Could you check a few things on this model? Use its own coordinates, in mm. A direction names the side the tool comes from. Coordinates: 2 decimals unless noted, no trailing zeros. Write each loop counter-clockwise with the first axis right and the second up, starting at its lowest first coordinate (ties: lowest second). Pieces come first, ordered by that corner, then holes.
```python
from build123d import *

# Parameters (mm, degrees)
EXTRUDE_1_DEPTH             = 90
SKETCH_2_W                  = 90
SKETCH_2_H                  = 17.75
EXTRUDE_2_DEPTH             = 8.2
SKETCH_3_W                  = 90
SKETCH_3_H                  = 50.95
EXTRUDE_3_DEPTH             = 8.2
SKETCH_4_W                  = 3.95
SKETCH_4_H                  = 29.5
CUT_EXTRUDE_1_DEPTH         = 96.44153315
SKETCH_5_W                  = 3.95
SKETCH_5_H                  = 6.2
CUT_EXTRUDE_2_DEPTH         = 96.44153315
SKETCH_6_W                  = 2.25
SKETCH_6_H                  = 3.95
CUT_EXTRUDE_3_DEPTH         = 96.44153315
SKETCH_7_W                  = 4.5
SKETCH_7_H                  = 3.95
CUT_EXTRUDE_4_DEPTH         = 96.44153315
SKETCH_8_W                  = 2.25
SKETCH_8_H                  = 3.95
CUT_EXTRUDE_5_DEPTH         = 96.44153315
SKETCH_9_W                  = 3.95
SKETCH_9_H                  = 2.25
CUT_EXTRUDE_6_DEPTH         = 96.44153315
SKETCH_10_W                 = 20.2
SKETCH_10_H                 = 45.2
CUT_EXTRUDE_7_DEPTH         = 86
HOLE_WIZARD_2_5_2_5_1_D     = 2.5
HOLE_WIZARD_4_5_4_5_1_D     = 4.5
HOLE_WIZARD_8_3_8_3_1_D     = 8.3
HOLE_WIZARD_8_3_8_3_1_DEPTH = 3.2
FILLET_1_R                  = 2
FILLET_2_R                  = 2
EXTRUDE_START               = -90
SKETCH_17_R                 = 1.25
EXTRUDE_4_DEPTH             = 90
CUT_EXTRUDE_START           = -100
SKETCH_18_R                 = 4.15
CUT_EXTRUDE_8_DEPTH         = 100


with BuildPart() as part:
    # Эскиз1 → Бобышка-Вытянуть1 (new body)
    with BuildSketch(Plane(origin=(90, 0, 0), x_dir=(0, 0, -1), z_dir=(1, 0, 0))):
        with BuildLine():
            Line((6.75, -24.093761792), (6.75, 19.25))
            Line((6.75, 19.25), (-11.593761792, 19.25))
            ThreePointArc((-11.593761792, 19.25), (-15.325, 18), (-11.593761792, 16.75))
            Line((-11.593761792, 16.75), (-11, 16.75))
            Line((-11, 16.75), (-11, -16.75))
            Line((-11, -16.75), (-11.593761792, -16.75))
            ThreePointArc((-11.593761792, -16.75), (-15.325, -18), (-11.593761792, -19.25))
            Line((-11.593761792, -19.25), (-11, -19.25))
            Line((-11, -19.25), (-11, -23.5))
            Line((-11, -23.5), (-6.75, -23.5))
            Line((-6.75, -23.5), (-6.75, -24.093761792))
            ThreePointArc((-6.75, -24.093761792), (-5.5, -27.825), (-4.25, -24.093761792))
            Line((-4.25, -24.093761792), (-4.25, -23.5))
            Line((-4.25, -23.5), (4.25, -23.5))
            Line((4.25, -23.5), (4.25, -24.093761792))
            ThreePointArc((4.25, -24.093761792), (5.5, -27.825), (6.75, -24.093761792))
        make_face()
    extrude(amount=-EXTRUDE_1_DEPTH)

    # Эскиз2 → Бобышка-Вытянуть2 (add)
    with BuildSketch(Plane(origin=(0, 19.25, 0), x_dir=(-1, 0, 0), z_dir=(0, 1, 0))):
        with Locations((-45, 2.125)):
            Rectangle(SKETCH_2_W, SKETCH_2_H)
    extrude(amount=EXTRUDE_2_DEPTH)

    # Эскиз3 → Бобышка-Вытянуть3 (add)
    with BuildSketch(Plane(origin=(0, 0, -6.75), x_dir=(-1, 0, 0), z_dir=(0, 0, -1))):
        with Locations((-45, 1.975)):
            Rectangle(SKETCH_3_W, SKETCH_3_H)
    extrude(amount=EXTRUDE_3_DEPTH)

    # Эскиз4 → Вырез-Вытянуть1 (cut, through all)
    with BuildSketch(Plane.ZY):
        with Locations((-12.975, 0)):
            Rectangle(SKETCH_4_W, SKETCH_4_H)
    extrude(amount=-CUT_EXTRUDE_1_DEPTH, mode=Mode.SUBTRACT)

    # Эскиз5 → Вырез-Вытянуть2 (cut, through all)
    with BuildSketch(Plane.ZY):
        with Locations((-12.975, 24.35)):
            Rectangle(SKETCH_5_W, SKETCH_5_H)
    extrude(amount=-CUT_EXTRUDE_2_DEPTH, mode=Mode.SUBTRACT)

    # Эскиз6 → Вырез-Вытянуть3 (cut, through all)
    with BuildSketch(Plane.ZY):
        with Locations((-9.875, 25.475)):
            Rectangle(SKETCH_6_W, SKETCH_6_H)
    extrude(amount=-CUT_EXTRUDE_3_DEPTH, mode=Mode.SUBTRACT)

    # Эскиз7 → Вырез-Вытянуть4 (cut, through all)
    with BuildSketch(Plane.ZY):
        with Locations((0, 25.475)):
            Rectangle(SKETCH_7_W, SKETCH_7_H)
    extrude(amount=-CUT_EXTRUDE_4_DEPTH, mode=Mode.SUBTRACT)

    # Эскиз8 → Вырез-Вытянуть5 (cut, through all)
    with BuildSketch(Plane.ZY):
        with Locations((9.875, 25.475)):
            Rectangle(SKETCH_8_W, SKETCH_8_H)
    extrude(amount=-CUT_EXTRUDE_5_DEPTH, mode=Mode.SUBTRACT)

    # Эскиз9 → Вырез-Вытянуть6 (cut, through all)
    with BuildSketch(Plane.ZY):
        with Locations((-12.975, -22.375)):
            Rectangle(SKETCH_9_W, SKETCH_9_H)
    extrude(amount=-CUT_EXTRUDE_6_DEPTH, mode=Mode.SUBTRACT)

    # Эскиз10 → Вырез-Вытянуть7 (cut)
    with BuildSketch(Plane(origin=(90, 0, 0), x_dir=(0, 0, -1), z_dir=(1, 0, 0))):
        Rectangle(SKETCH_10_W, SKETCH_10_H)
    extrude(amount=-CUT_EXTRUDE_7_DEPTH, mode=Mode.SUBTRACT)

    # Диаметр отверстия Ø2.5 (2.5)1 (through all)
    with Locations(Plane(origin=(90, 0, 0), x_dir=(0, 0, -1), z_dir=(1, 0, 0))):
        with Locations((5.5, -25.75), (-13.25, -18), (-5.5, -25.75), (-13.25, 18)):
            Hole(HOLE_WIZARD_2_5_2_5_1_D / 2)

    # Диаметр отверстия Ø4.5 (4.5)1 (through all)
    with Locations(Plane.ZY):
        with Locations((-13.25, -18), (-13.25, 18), (-5.5, 25.75), (5.5, 25.75)):
            Hole(HOLE_WIZARD_4_5_4_5_1_D / 2)

    # Диаметр отверстия Ø8.3 (8.3)1
    with Locations(Plane.ZY):
        with Locations((0, 0)):
            Hole(HOLE_WIZARD_8_3_8_3_1_D / 2, depth=HOLE_WIZARD_8_3_8_3_1_DEPTH)

    # Скругление1
    fillet_1_edges = [part.edges().sort_by_distance(p)[0] for p in [
        (45, 23.5, 8.75),
    ]]
    fillet(fillet_1_edges, radius=FILLET_1_R)

    # Скругление2
    fillet_2_edges = [part.edges().sort_by_distance(p)[0] for p in [
        (45, 23.5, -8.75),
        (45, 23.5, 2.25),
        (45, 23.5, -2.25),
        (45, -21.25, -11),
        (4, 0, -10.1),
        (4, -22.6, 0),
        (4, 0, 10.1),
        (4, 22.6, 0),
        (45, 14.75, -11),
        (45, -14.75, -11),
        (45, 21.25, -11),
    ]]
    fillet(fillet_2_edges, radius=FILLET_2_R)

    # Эскиз17 → Бобышка-Вытянуть4 (add)
    with BuildSketch(Plane(origin=(90, 0, 0), x_dir=(0, 0, -1), z_dir=(1, 0, 0)).offset(EXTRUDE_START)):
        with Locations((5.5, -25.75)):
            Circle(SKETCH_17_R)
        with Locations((-5.5, -25.75)):
            Circle(SKETCH_17_R)
        with Locations((-13.25, -18)):
            Circle(SKETCH_17_R)
        with Locations((-13.25, 18)):
            Circle(SKETCH_17_R)
    extrude(amount=EXTRUDE_4_DEPTH)

    # Эскиз18 → Вырез-Вытянуть8 (cut)
    with BuildSketch(Plane.ZY.offset(CUT_EXTRUDE_START)):
        Circle(SKETCH_18_R)
    extrude(amount=CUT_EXTRUDE_8_DEPTH, mode=Mode.SUBTRACT)


solid = part.part
```
1. I want a section at D-D on y = -6. Please give me the cut outline in (x, z), plus the area to 3 significant figures.
Verdict:
outline: (0, -11) - (90, -11) - (90, -10.1) - (6, -10.1) arc R2 cw to (4, -8.1) - (4, 8.1) arc R2 cw to (6, 10.1) - (90, 10.1) - (90, 11) - (0, 11) - close
area: 245 mm2
2. On a 3-axis mill with a long thin cutter (end or side, diameter ignored), from which of +Z, -Z, +X, -X, +Y, -Y can I reach the whole of each face in a straight line? I mean faces 1 (the face through (44, 26, -2.25)), 2 (the face through (45.63, 14.18, -11.6)), 3 (the face through (44, 26, 8.75)). Say none if no direction works.
Verdict:
face 1: +X, -X, +Y
face 2: -Z, +X, -X
face 3: +Z, +X, -X, +Y
3. I want a section at C-C on z = -5.5. Please give me the cut outline in (x, y) (3 decimals), plus the area to 3 significant figures.
Verdict:
outline: (0, -27.825) - (90, -27.825) - (90, -22.6) - (6, -22.6) arc R2 cw to (4, -20.6) - (4, 20.6) arc R2 cw to (6, 22.6) - (90, 22.6) - (90, 23.5) - (0, 23.5) - close
area: 734 mm2
4. For pin 1 (1.6 mm diameter, centred on x = 36, y = 26, fed in from -Z); pin 2 (0.7 mm diameter, centred on x = 40, z = 11.5, fed in from +Y); pin 3 (1 mm diameter, centred on x = 25.5, y = 26.5, fed in from +Z), each with a flat end and sliding along its axis, tell me the tip position at first contact or that it passes through.
Verdict:
pin 1: stops at z = -8.77
pin 2: stops at y = 19.53
pin 3: stops at z = 8.75
5. I want a section at B-B on y = -25.75. Please give me the cut outline in (x, z) (3 decimals).
Verdict:
outline: (0, -7.575) - (90, -7.575) - (90, -3.425) - (0, -3.425) - close; (0, 3.425) - (90, 3.425) - (90, 7.575) - (0, 7.575) - close
6. Please list where these lines run through material, in increasing order: line 1 along Z through (x, y) = (51, 25.75); line 2 along Y through (x, z) = (28, -13.25).
Verdict:
line 1: z = -8.75 to -7.75, -3.25 to -2.25, 2.25 to 3.25, 7.75 to 8.75
line 2: y = -21.25 to -20.25, -15.75 to -14.75, 14.75 to 15.75, 20.25 to 21.25
7. I want a section at A-A on z = 13.25. Please give me the cut outline in (x, y) (3 decimals).
Verdict:
outline: (0, -20.075) - (90, -20.075) - (90, -15.925) - (0, -15.925) - close; (0, 15.925) - (90, 15.925) - (90, 20.075) - (0, 20.075) - close
